```python
from build123d import *

# Parameters (mm, degrees)
F0_W     = 40
F0_H     = 35.319249
F1_DEPTH = 7.5
F2_W     = 36
F2_H     = 31.319249
F3_DEPTH = 3.5
F4_R     = 4
F5_DEPTH = 10


with BuildPart() as f1:
    # F0 (on Front) → F1 (new body, symmetric)
    with BuildSketch(Plane.XZ):
        with Locations((20, 17.659624)):
            Rectangle(F0_W, F0_H)
    extrude(amount=F1_DEPTH, both=True)

    # F2 (on Front) → F3 (cut, symmetric)
    with BuildSketch(Plane.XZ):
        with Locations((22, 19.659624)):
            Rectangle(F2_W, F2_H)
    extrude(amount=F3_DEPTH, both=True, mode=Mode.SUBTRACT)

    # F4 (on face) → F5 (join)
    with BuildSketch(Plane(origin=(0, 0, 0), x_dir=(1, 0, 0), z_dir=(0, 0, -1))):
        with Locations((8, 0)):
            Circle(F4_R)
    extrude(amount=F5_DEPTH)


solid = f1.part
```
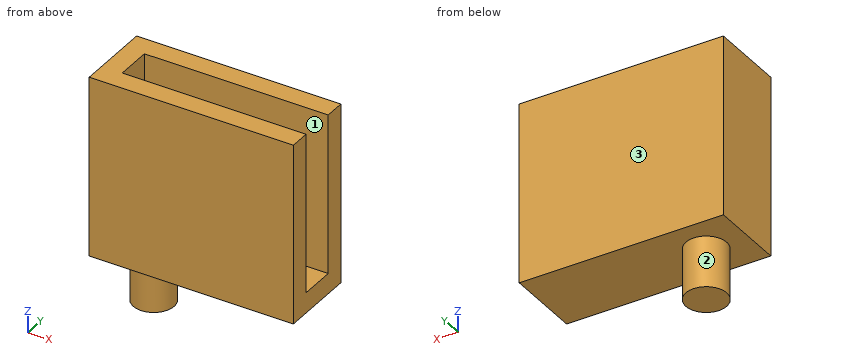
Input: part model. Units: mm. Frame: model coordinates. Face numbers are marked on the shaded views. Give positions to 0.01 mm unless a question says otherwise; leave off trailing zeros. Loops run counter-clockwise (first coordinate to the right, second up) from the corner with the lowest first, then second, coordinate; pieces in that order, holes last.
1) Section query D-D on x = 23. Return the cut outline in (y, z).
A:
outline: (-7.5, 0) - (7.5, 0) - (7.5, 35.32) - (3.5, 35.32) - (3.5, 4) - (-3.5, 4) - (-3.5, 35.32) - (-7.5, 35.32) - close
2) Line query: L1, parallel to Y at x = 19, z = 23.5; L2, parallel to Z at x = 2, y = 4; L3, parallel to X at y = 3, z = 24. Output: solid intervals per line, ascending.
A:
L1: y = -7.5 to -3.5, 3.5 to 7.5
L2: z = 0 to 35.32
L3: x = 0 to 4
3) Section query C-C on y = 0. Return the cut outline in (x, z).
A:
outline: (0, 0) - (4, 0) - (4, -10) - (12, -10) - (12, 0) - (40, 0) - (40, 4) - (4, 4) - (4, 35.32) - (0, 35.32) - close
4) Section query A-A on z = 29.5. Return the cut outline in (x, y).
A:
outline: (0, -7.5) - (40, -7.5) - (40, -3.5) - (4, -3.5) - (4, 3.5) - (40, 3.5) - (40, 7.5) - (0, 7.5) - close
5) Section query B-B on x = 8. Return the cut outline in (y, z).
A:
outline: (-7.5, 0) - (-4, 0) - (-4, -10) - (4, -10) - (4, 0) - (7.5, 0) - (7.5, 35.32) - (3.5, 35.32) - (3.5, 4) - (-3.5, 4) - (-3.5, 35.32) - (-7.5, 35.32) - close
6) Mould query, pull axis Y, two halves, no side actions, for the marked faces 1, 2 and 3. Classes: released by +Y, released by -Y, zero draft, split by the parting line, or undercut.
A:
face 1: undercut
face 2: split by the parting line
face 3: released by +Y
7) Contact query for flat-ended pins moving along their axis: pin 1 (3.5 mm diameter, centred on y = 0.5, z = 13, fed in from +X); pin 2 (5 mm diameter, centred on y = 1, z = -5, fed in from -X); pin 3 (1.5 mm diameter, centred on y = 3.5, z = -4, fed in from -X). Output: stop coordinate, or through.
A:
pin 1: stops at x = 4
pin 2: stops at x = 4
pin 3: stops at x = 5.1
